Model file for the job. Use its own axes, mm. A direction names the side the tool comes from. Give positions to 0.01 mm unless a question says otherwise; leave off trailing zeros. Write each loop counter-clockwise with the first axis right and the second up, starting at its lowest first coordinate (ties: lowest second). Pieces come first, ordered by that corner, then holes. Notation, with made-up numbers: (72, -13.5) - (90, -13.5) arc R14 cw to (90, 3.5) - close; hole circle Ø10 at (37, -35). An arc over 180 degrees is marked (long way). Use a Markdown table: item, result. Add a question column.
```python
from build123d import *

# Parameters (mm, degrees)
MODEL_R             = 11.05
MODEL_R_2           = 2
MODEL_R_3           = 3.5
MODEL_W             = 15.4
MODEL_H             = 5.4
MODEL_W_2           = 5
MODEL_H_2           = 15
BOSS_EXTRUDE1_DEPTH = 17


with BuildPart() as part:
    # Model → Boss-Extrude1 (new body)
    with BuildSketch(Plane.XY):
        with BuildLine():
            Line((-158.978150708, -561.169218198), (-164.178150708, -561.169218198))
            Line((-164.178150708, -561.169218198), (-164.178150708, -628.419218198))
            Line((-164.178150708, -628.419218198), (-158.978150708, -628.419218198))
            Line((-158.978150708, -628.419218198), (-158.978150708, -653.619218198))
            Line((-158.978150708, -653.619218198), (-164.178150708, -653.619218198))
            Line((-164.178150708, -653.619218198), (-164.178150708, -673.619218198))
            Line((-164.178150708, -673.619218198), (-158.978150708, -673.619218198))
            Line((-158.978150708, -673.619218198), (-158.978150708, -693.619218198))
            Line((-158.978150708, -693.619218198), (-164.178150708, -693.619218198))
            Line((-164.178150708, -693.619218198), (-164.178150708, -713.619218198))
            Line((-164.178150708, -713.619218198), (-158.978150708, -713.619218198))
            Line((-158.978150708, -713.619218198), (-158.978150708, -733.619218198))
            Line((-158.978150708, -733.619218198), (-164.178150708, -733.619218198))
            Line((-164.178150708, -733.619218198), (-164.178150708, -758.619218198))
            Line((-164.178150708, -758.619218198), (-158.978150708, -758.619218198))
            Line((-158.978150708, -758.619218198), (-158.978150708, -778.819218198))
            Line((-158.978150708, -778.819218198), (-164.178150708, -778.819218198))
            Line((-164.178150708, -778.819218198), (-164.178150708, -798.619218198))
            ThreePointArc((-164.178150708, -798.619218198), (-152.462421956, -826.903489445), (-124.178150708, -838.619218198))
            Line((-124.178150708, -838.619218198), (135.821849292, -838.619218198))
            ThreePointArc((135.821849292, -838.619218198), (164.106120539, -826.903489445), (175.821849292, -798.619218198))
            Line((175.821849292, -798.619218198), (175.821849292, -498.469218198))
            Line((175.821849292, -498.469218198), (138.321849292, -498.469218198))
            Line((138.321849292, -498.469218198), (138.321849292, -503.669218198))
            Line((138.321849292, -503.669218198), (108.321849292, -503.669218198))
            Line((108.321849292, -503.669218198), (108.321849292, -498.469218198))
            Line((108.321849292, -498.469218198), (78.321849292, -498.469218198))
            Line((78.321849292, -498.469218198), (78.321849292, -503.669218198))
            Line((78.321849292, -503.669218198), (48.321849292, -503.669218198))
            Line((48.321849292, -503.669218198), (48.321849292, -498.469218198))
            Line((48.321849292, -498.469218198), (18.321849292, -498.469218198))
            Line((18.321849292, -498.469218198), (18.321849292, -503.669218198))
            Line((18.321849292, -503.669218198), (-11.678150708, -503.669218198))
            Line((-11.678150708, -503.669218198), (-11.678150708, -498.469218198))
            Line((-11.678150708, -498.469218198), (-41.678150708, -498.469218198))
            Line((-41.678150708, -498.469218198), (-41.678150708, -503.669218198))
            Line((-41.678150708, -503.669218198), (-71.678150708, -503.669218198))
            Line((-71.678150708, -503.669218198), (-71.678150708, -498.469218198))
            Line((-71.678150708, -498.469218198), (-101.678150708, -498.469218198))
            Line((-101.678150708, -498.469218198), (-101.678150708, -503.669218198))
            Line((-101.678150708, -503.669218198), (-131.678150708, -503.669218198))
            Line((-131.678150708, -503.669218198), (-131.678150708, -498.469218198))
            Line((-131.678150708, -498.469218198), (-146.678150708, -498.469218198))
            Line((-146.678150708, -498.469218198), (-146.678150708, -503.469218198))
            Line((-146.678150708, -503.469218198), (-159.178150708, -515.969218198))
            Line((-159.178150708, -515.969218198), (-164.178150708, -515.969218198))
            Line((-164.178150708, -515.969218198), (-164.178150708, -530.969218198))
            Line((-164.178150708, -530.969218198), (-158.978150708, -530.969218198))
            Line((-158.978150708, -530.969218198), (-158.978150708, -561.169218198))
        make_face()
        with Locations((86.821849292, -767.469218198)):
            Circle(MODEL_R, mode=Mode.SUBTRACT)
        with Locations((-139.178150708, -561.469218198)):
            Circle(MODEL_R, mode=Mode.SUBTRACT)
        with Locations((-79.178150708, -813.619218198)):
            Circle(MODEL_R_2, mode=Mode.SUBTRACT)
        with Locations((-139.178150708, -746.469218198)):
            Circle(MODEL_R_3, mode=Mode.SUBTRACT)
        with Locations((-139.178150708, -761.469218198)):
            Circle(MODEL_R_3, mode=Mode.SUBTRACT)
        with BuildLine():
            Line((60.821849292, -613.469218198), (60.821849292, -563.469218198))
            ThreePointArc((60.821849292, -563.469218198), (5.821849292, -508.469218198), (-49.178150708, -563.469218198))
            Line((-49.178150708, -563.469218198), (-49.178150708, -613.469218198))
            ThreePointArc((-49.178150708, -613.469218198), (-37.462421956, -641.753489445), (-9.178150708, -653.469218198))
            Line((-9.178150708, -653.469218198), (20.821849292, -653.469218198))
            ThreePointArc((20.821849292, -653.469218198), (49.106120539, -641.753489445), (60.821849292, -613.469218198))
        make_face(mode=Mode.SUBTRACT)
        with Locations((-136.678150708, -631.119218198)):
            Rectangle(MODEL_W, MODEL_H, mode=Mode.SUBTRACT)
        with Locations((-136.678150708, -776.119218198)):
            Rectangle(MODEL_W, MODEL_H, mode=Mode.SUBTRACT)
        with Locations((73.321849292, -523.969218198)):
            Rectangle(MODEL_W_2, MODEL_H_2, mode=Mode.SUBTRACT)
        with Locations((168.321849292, -535.969218198)):
            Rectangle(MODEL_W_2, MODEL_H_2, mode=Mode.SUBTRACT)
        with Locations((-61.678150708, -523.969218198)):
            Rectangle(MODEL_W_2, MODEL_H_2, mode=Mode.SUBTRACT)
    extrude(amount=BOSS_EXTRUDE1_DEPTH)


solid = part.part
```
(1) Band-saw the part on C-C (x = 66.5). Write the cut outline in (y, z).
(2) Two-plate mould, pull along X, no slides. Class faces 5 (the flat face through (-164.178, -703, 8)), 6 (the flat face through (157, -498.469, 8)), 7 (the flat face through (4, -503.669, 8)): +X half, -X half, draft (parallel to the pull), parting line (faces both ways), or undercut.
(3) Flat gauge pins, fed straight in: pin 1 (4 mm diameter, centred on x = -161, z = 4.5, fed in from -Y); pin 2 (4 mm diameter, centred on y = -502, z = 5.5, fed in from -X); pin 3 (1.6 mm diameter, centred on x = -162.5, z = 6, fed in from +Y). Where does each tip first touch, or does it go through?
(4) Band-saw the part on A-A (y = -602). Write the cut outline in (x, z).
(5) Band-saw the part on D-D (y = -689). Write the cut outline in (x, z), then the cut area to 3 significant figures.
(6) Probe probe 1 along X at (y, z) = (-591.5, 3); probe 2 along X at (y, z) = (-518, 6.5); probe 3 along Y at (x, z) = (116.5, 11). List the from-to ranges inside material, lowest first. Write a range as [from, to].
(7) Which spindle directions (+Z, -Z, +X, -X, +Y, -Y) get a long thin tool onto all of the face, cutting with end or side? Do faces 1 (the flat face through (-158.978, -641, 8)), 2 (the flat face through (-137, -628.419, 8)), 3 (the flat face through (-86, -498.469, 8)), 4 (the flat face through (124, -503.669, 8)). Say none if no direction does.
(8) Band-saw the part on B-B (x = 4). Write the cut outline in (y, z), then the cut area to 3 significant figures.
Model answer:
| question | item | result |
|---|---|---|
| 1 | outline | (-838.62, 0) - (-503.67, 0) - (-503.67, 17) - (-838.62, 17) - close |
| 2 | face 5 | -X half |
| 2 | face 6 | draft |
| 2 | face 7 | undercut |
| 3 | pin 1 | stops at y = -818.3 |
| 3 | pin 2 | stops at x = -147.21 |
| 3 | pin 3 | stops at y = -515.97 |
| 4 | outline | (-164.18, 0) - (-49.18, 0) - (-49.18, 17) - (-164.18, 17) - close; (60.82, 0) - (175.82, 0) - (175.82, 17) - (60.82, 17) - close |
| 5 | outline | (-158.98, 0) - (175.82, 0) - (175.82, 17) - (-158.98, 17) - close |
| 5 | area | 5,690 mm^2 |
| 6 | probe 1 | x = [-164.18, -49.18], [60.82, 175.82] |
| 6 | probe 2 | x = [-164.18, -64.18], [-59.18, -25.12], [36.77, 70.82], [75.82, 175.82] |
| 6 | probe 3 | y = [-838.62, -503.67] |
| 7 | face 1 | +Z, -Z, -X |
| 7 | face 2 | +Z, -Z |
| 7 | face 3 | +Z, -Z, +X, -X, +Y |
| 7 | face 4 | +Z, -Z, +Y |
| 8 | outline | (-838.62, 0) - (-653.47, 0) - (-653.47, 17) - (-838.62, 17) - close; (-508.5, 0) - (-503.67, 0) - (-503.67, 17) - (-508.5, 17) - close |
| 8 | area | 3,230 mm^2 |
